For this review, take the finished solid that the model builds, in its own axes (mm). A direction names the side the tool comes from. Round coordinates to 2 decimals unless told otherwise and drop trailing zeros. Write each loop counter-clockwise with the first axis right and the second up, starting at its lowest first coordinate (ties: lowest second). Pieces come first, ordered by that corner, then holes.
from build123d import *

# Parameters (mm, degrees)
F2_R = 5.08


with BuildPart() as f1:
    # F0 (on Front) → F1 (revolve)
    with BuildSketch(Plane.XZ):
        with BuildLine():
            Line((-38.1, 0), (0, 0))
            Line((0, 0), (0, 168.402))
            Line((0, 168.402), (-17.877694, 168.402))
            Line((-17.877694, 168.402), (-17.877694, 158.566087))
            Line((-17.877694, 158.566087), (-14.2875, 158.566087))
            Line((-14.2875, 158.566087), (-14.2875, 151.651561))
            ThreePointArc((-14.2875, 151.651561), (-31.12548, 144.677041), (-38.1, 127.839061))
            Line((-38.1, 127.839061), (-38.1, 0))
        make_face()
    revolve(axis=Axis((0, 0, 84.201), (0, 0, 1)))

    # F2
    f2_edges = [f1.edges().sort_by_distance(p)[0] for p in [
        (38.1, 0, 0),
    ]]
    fillet(f2_edges, radius=F2_R)


solid = f1.part
(1) For faces 1 (the face through (30.235, 23.183, 65.6)), 2 (the face through (17.86, -0.79, 163.42)), 3 (the face through (14.274, -0.628, 155.06)), list the 3-axis set-ups (+Z, -Z, +X, -X, +Y, -Y) from which the entire face can be reached by the end or side of a thin tool; tool diameter is ignored.
Geometry check:
face 1: +Z, -Z
face 2: +Z
face 3: none
(2) For pin 1 Ø10.5 at (x, y) = (5.5, 5) entering from -Z; pin 2 Ø12 at (y, z) = (-4, 135.5) entering from +X; pin 3 Ø12 at (x, z) = (3, 37.5) entering from -Y; pin 4 Ø1.5 at (x, z) = (23.5, 85) entering from -Y, all flat-tipped, find the tip position at first contact; note any pin that passes through.
Geometry check:
pin 1: stops at z = 0
pin 2: stops at x = 37.97
pin 3: stops at y = -38.1
pin 4: stops at y = -30.56
(3) For line 1 along Z through (x, y) = (-0.5, -15.5); line 2 along X through (y, z) = (1, 54); line 3 along Z through (x, y) = (14, 19), list the stretches that pass through material, from the lowest coordinate up.
Geometry check:
line 1: z = 0 to 151.62, 158.57 to 168.4
line 2: x = -38.09 to 38.09
line 3: z = 0 to 149.75
(4) We need section A-A, the plane z = 107.5. Give the boundary of the cut face in (x, y), and give its area (3 significant figures).
Geometry check:
outline: circle Ø76.2 at (0, 0)
area: 4,560 mm2
